Part model, mm, in its own coordinate system. Coordinates: 2 decimals unless noted, no trailing zeros. Loops run counter-clockwise (first coordinate to the right, second up) from the corner with the lowest first, then second, coordinate; pieces in that order, holes last.
```python
from build123d import *

# Parameters (mm, degrees)
F0_W     = 304.8
F0_H     = 158.75
F0_R     = 12.7
F0_R_2   = 50.8
F1_DEPTH = 19.05
F2_SIZE2 = 7.890758
F2_SIZE  = 19.04999


# Not quite as in the source:
# - a fillet or chamfer is up to 0.001 mm smaller than in the source, because OpenCascade refuses the exact size


with BuildPart() as f1:
    # F0 (on Top) → F1 (new body)
    with BuildSketch(Plane.XY):
        Rectangle(F0_W, F0_H)
        with Locations((-88.9, 0)):
            Circle(F0_R, mode=Mode.SUBTRACT)
        Circle(F0_R_2, mode=Mode.SUBTRACT)
        with BuildLine():
            ThreePointArc((88.9, -12.7), (79.9197438789, 8.9802561211), (101.6, 0))
            ThreePointArc((101.6, 0), (97.8802561211, -8.9802561211), (88.9, -12.7))
        make_face(mode=Mode.SUBTRACT)
    extrude(amount=F1_DEPTH)

    # F2 (size 19.05 and 7.8907683632 in the source; OpenCascade refuses exactly that, so slightly less here)
    f2_edges = [f1.edges().sort_by_distance(p)[0] for p in [
        (0, 79.375, 19.05),
    ]]
    f2_side = f1.faces().sort_by_distance((0, 79.375, 9.525))[0]
    chamfer(f2_edges, length=F2_SIZE, length2=F2_SIZE2, reference=f2_side)


solid = f1.part
```
Q1. Probe line 1 (X direction, y = -6.5, z = 13.5); line 2 (Y direction, x = 77.5, z = 8) (3 decimals); line 3 (X direction, y = -42, z = 11). List the from-to ranges inside material, lowest first.
Q2. Mould opens along X. For faces 1 (the flat face through (-152.4, -1, 9)), 2 (the cylindrical face through (-76.786, 3.815, 9.392)), 3 (the flat face through (-2, -79.375, 9)) say: released by +X, released by -X, zero draft, split by the parting line, or undercut.
Q3. Saw through at C-C (z = 13.75). List the corners of the cut face in (x, y) (3 decimals), plus the area to 3 significant figures.
Q4. Saw through at B-B (y = 33). List the corners of the cut face in (x, z), plus the area to 3 significant figures.
Q5. Drop flat-ended pins along their axis: P1, Ø1.5, axis at x = 77, z = 7.5, coming from the +Y side; P2, Ø5, axis at x = -21.5, z = 11.5, coming from the +Y side; P3, Ø15, axis at x = 88.9, y = 0, coming from the +Z side. Give the stop position or say it passes through.
Checked values:
1. line 1: x = -152.4 to -99.81, -77.99 to -50.38, 50.38 to 77.99, 99.81 to 152.4
1. line 2: y = -79.375 to -5.597, 5.597 to 76.061
1. line 3: x = -152.4 to -28.58, 28.58 to 152.4
2. face 1: released by -X
2. face 2: undercut
2. face 3: zero draft
3. outline: (-152.4, -79.375) - (152.4, -79.375) - (152.4, 73.68) - (-152.4, 73.68) - close; hole circle Ø25.4 at (-88.9, 0); hole circle Ø101.6 at (0, 0); hole circle Ø25.4 at (88.9, 0)
3. area: 37,500 mm2
4. outline: (-152.4, 0) - (-38.62, 0) - (-38.62, 19.05) - (-152.4, 19.05) - close; (38.62, 0) - (152.4, 0) - (152.4, 19.05) - (38.62, 19.05) - close
4. area: 4,330 mm2
5. P1: stops at y = 76.58
5. P2: stops at y = 75.65
5. P3: passes through
